```python
from build123d import *

# Parameters (mm, degrees)
SKETCH3_R           = 4.445
SKETCH3_R_2         = 1.2573
BOSS_EXTRUDE1_DEPTH = 1.778
BOSS_EXTRUDE2_DEPTH = 1.778
CIRPATTERN1_COUNT   = 5


with BuildPart() as part:
    # Sketch1 → Revolve1 (revolve)
    with BuildSketch(Plane.XY):
        with BuildLine():
            Line((-1.778, 48.26), (1.778, 48.26))
            Line((1.778, 48.26), (1.778, 53.34))
            ThreePointArc((1.778, 53.34), (0, 51.562), (-1.778, 53.34))
            Line((-1.778, 53.34), (-1.778, 48.26))
        make_face()
    revolve(axis=Axis((0, 0, 0), (-1, 0, 0)))



with BuildPart() as body_2:
    # Sketch3 → Boss-Extrude1 (new body, symmetric)
    with BuildSketch(Plane(origin=(0, 0, 0), x_dir=(0, 0, -1), z_dir=(1, 0, 0))):
        Circle(SKETCH3_R)
        Circle(SKETCH3_R_2, mode=Mode.SUBTRACT)
    extrude(amount=BOSS_EXTRUDE1_DEPTH, both=True)


with BuildPart() as part_1:
    add(part.part)

    add(body_2.part)  # Boss-Extrude2 merges body 2
    # Sketch4 → Boss-Extrude2 (add, symmetric)
    with BuildSketch(Plane(origin=(0, 0, 0), x_dir=(0, 0, -1), z_dir=(1, 0, 0))):
        with BuildLine():
            add(Edge.make_bspline(
                [(4.238371501, 1.339489461), (-0.797084769, 33.68038201), (-5.741030131, 43.234836537), (-16.711740024, 45.274113413)],
                knots=[0.007862153, 0.007862153, 0.007862153, 0.007862153, 0.582841342, 0.582841342, 0.582841342, 0.582841342], degree=3))
            ThreePointArc((-16.711740024, 45.274113413), (-22.926461421, 42.466515829), (-28.683393703, 38.810958835))
            add(Edge.make_bspline(
                [(2.269041799, 3.822234204), (-8.332097903, 29.7473311), (-28.683393703, 38.810958835)],
                knots=[0, 0, 0, 0.658247548, 0.658247548, 0.658247548], degree=2))
            ThreePointArc((2.269041799, 3.822234204), (3.482472158, 2.76232016), (4.238371501, 1.339489461))
        make_face()
    boss_extrude2 = extrude(amount=BOSS_EXTRUDE2_DEPTH, both=True)

    # CirPattern1: Boss-Extrude2 ×5 about axis
    cirpattern1_axis = Axis((0, 0, 0), (1, 0, 0))
    for i in range(1, CIRPATTERN1_COUNT):
        add(boss_extrude2.rotate(cirpattern1_axis, i * 360 / CIRPATTERN1_COUNT))


solid = part_1.part
```
Geometry check sheet. Reference: the model listing, model coordinates, mm. Give positions to 0.01 mm unless a question says otherwise; leave off trailing zeros. Write item = value, one per line. Start each with the question number.
1. Go/stop test with flat-tipped pins: P1, Ø1, axis at x = 0.5, z = 9.5, coming from the +Y side; P2, Ø5, axis at y = 22, z = -21.5, coming from the +X side; P3, Ø2, axis at x = -0.5, y = -2, coming from the -Z side; P4, Ø1, axis at x = 0.5, y = 4, coming from the +Z side. Record where each tip stops, or that it passes through.
2. Thickness scan on probe 1 along Z at (x, y) = (0.3, -21); probe 2 along Y at (x, z) = (0.45, -35.5); probe 3 along Y at (x, z) = (1.1, 22.5). Record the ranges inside material, lowest first.
3. Draft check along Z on faces 1 (the face through (1.778, 0, -4)), 2 (the face through (-0.02, -1.23, 0.27)). Enter one of: +Z half, -Z half, draft (parallel to the pull), parting line (faces both ways), or undercut.
4. Section check A-A, the plane z = -35. Give the number of separate pieces and of enclosed holes in the cut face, plus the area to 3 significant figures.
Values follow:
q1.P1 = 51
q1.P2 = 1.78
q1.P3 = -52.35
q1.P4 = 51.72
q2.probe_1 = -47.12 to -16.5, 6.58 to 14.45, 43.45 to 47.12
q2.probe_2 = -37.47 to -32.69, -28.3 to -15.65, 18.97 to 37.47
q2.probe_3 = -46.82 to -42.69, -0.4 to 7.16, 35.53 to 46.82
q3.face_1 = draft
q3.face_2 = undercut
q4.separate_pieces = 3
q4.enclosed_holes = 0
q4.area = 135 mm^2
